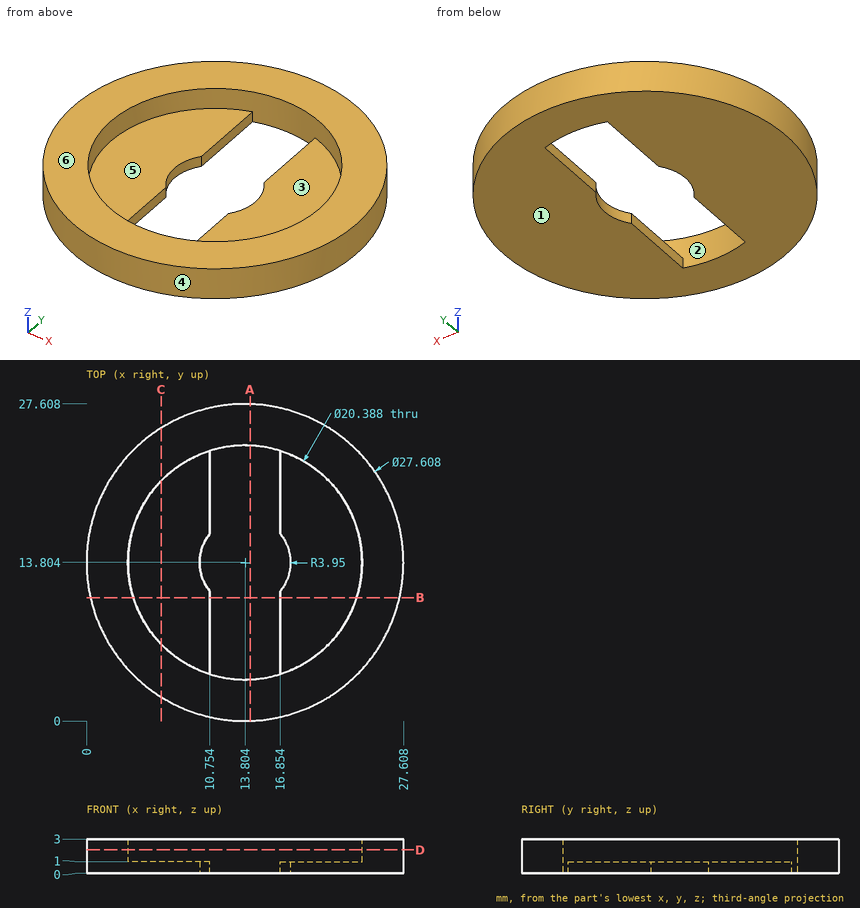
Answer from the drawing. Dimensions are ordinates in mm from the lowest x, y and z of the part. A direction names the side the tool comes from. Give positions to 0.01 mm unless a question says otherwise; leave off trailing zeros. Loops run counter-clockwise (first coordinate to the right, second up) from the corner with the lowest first, then second, coordinate; pieces in that order, holes last.
Item 1: The part is cut by section D-D (z = 2.05). Write down the section's boundary in (x, y), and give its area (3 significant figures).
Item 2: The mould has two halves that part along X. Classify the marked faces 1, 2, 3 and 4: released by +X, released by -X, zero draft, split by the parting line, or undercut.
Item 3: The part is cut by section C-C (x = 6.5). Write down the section's boundary in (y, z) (1 decimal).
Item 4: The part is cut by section A-A (x = 14.25). Write down the section's boundary in (y, z), and give its area (3 significant figures).
Item 5: Find the intervals of material crossed by line 1 along Y through (x, z) = (12, 2.05); line 2 along X through (y, z) = (11.25, 2.7) (1 decimal); line 3 along Y through (x, z) = (4.75, 1.8) (1 decimal), in increasing order.
Item 6: For the marked faces 5 and 6, determine the directions among +Z, -Z, +X, -X, +Y, -Y from which every point of the face is accessible in a straight line to the end or side of a thin tool.
Item 7: Each of these flat-tipped pins is pushed along its axis until it touches: pin 1 Ø1.1 at (y, z) = (8, 0.5) entering from +X; pin 2 Ø1.1 at (y, z) = (20.5, 0.5) entering from +X; pin 3 Ø3.5 at (x, y) = (21, 9.5) entering from +Z. Where does it stop, or does it pass through?
Item 8: The part is cut by section B-B (y = 10.75). Write down the section's boundary in (x, z) (1 decimal).
Taken from the geometry:
1. outline: circle Ø27.61 at (13.8, 13.8); hole circle Ø20.39 at (13.8, 13.8)
1. area: 272 mm2
2. face 1: zero draft
2. face 2: undercut
2. face 3: undercut
2. face 4: split by the parting line
3. outline: (2.1, 0) - (25.5, 0) - (25.5, 3) - (20.9, 3) - (20.9, 1) - (6.7, 1) - (6.7, 3) - (2.1, 3) - close
4. outline: (0.01, 0) - (3.62, 0) - (3.62, 3) - (0.01, 3) - close; (23.99, 0) - (27.6, 0) - (27.6, 3) - (23.99, 3) - close
4. area: 21.7 mm2
5. line 1: y = 0.12 to 3.77, 23.84 to 27.49
5. line 2: x = 0.2 to 3.9, 23.7 to 27.4
5. line 3: y = 3.4 to 9.1, 18.5 to 24.2
6. face 5: +Z
6. face 6: +Z, +X, -X, +Y, -Y
7. pin 1: stops at x = 26.57
7. pin 2: stops at x = 26.16
7. pin 3: stops at z = 1
8. outline: (0.3, 0) - (10.8, 0) - (10.8, 1) - (4.1, 1) - (4.1, 3) - (0.3, 3) - close; (16.9, 0) - (27.3, 0) - (27.3, 3) - (23.5, 3) - (23.5, 1) - (16.9, 1) - close
